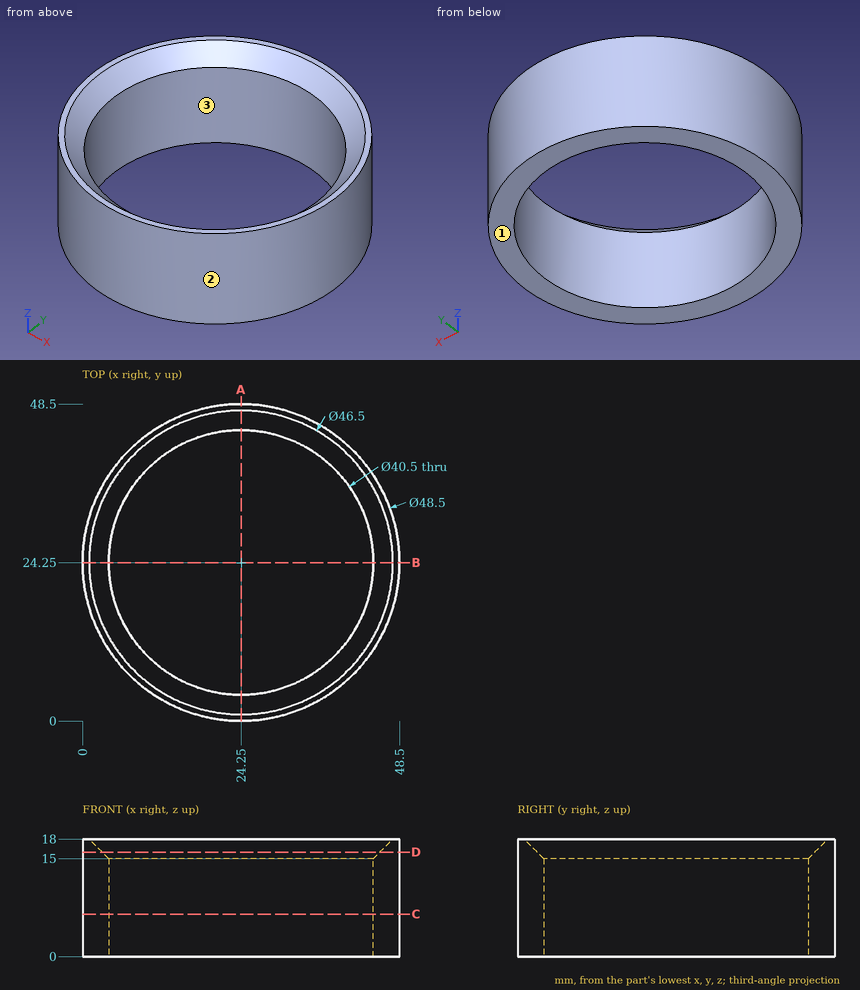
Drawing for the job (mm, zero at the part's lowest x, y, z). Give positions to 0.01 mm unless a question says otherwise; leave off trailing zeros. Order: outer loops, then holes, each group sorted by start corner. A loop starts at its lowest first (then second) coordinate and runs counter-clockwise, first axis right, second up. Notation, with made-up numbers: M -30,53.25 L 17,53.25 A3 cw 17,58.25 Z; hole C -38,29 d2. An arc over 180 degrees is marked long. Put each result on its own line as item: value. Start each with the question number.
(1) Saw through at C-C, the plane z = 6.5. Write the cut outline in (x, y).
(2) Drill centre lines: line 1 along Y through (x, z) = (24.25, 11.5); line 2 along X through (y, z) = (9.5, 4.5). Where is each one in solid material? Low to high.
(3) Flat gauge pins, fed straight in: pin 1 Ø10 at (y, z) = (43, 14) entering from -X (3 decimals); pin 2 Ø8 at (x, z) = (7, 2.5) entering from -Y; pin 3 Ø1 at (x, z) = (43.5, 10) entering from -Y. Where does each tip first touch, or does it go through?
(4) Saw through at D-D, the plane z = 16. Write the cut outline in (x, y).
(5) Saw through at A-A, the plane x = 24.25. Write the cut outline in (y, z).
(6) Mould opens along X. For the marked faces 1, 2 and 3 say: +X half, -X half, draft (parallel to the pull), parting line (faces both ways), or undercut.
Check result:
1. outline: C 24.25,24.25 d48.5; hole C 24.25,24.25 d40.5
2. line 1: y = 0 to 4, 44.5 to 48.5
2. line 2: x = 5 to 10.38, 38.12 to 43.5
3. pin 1: stops at x = 4.275
3. pin 2: stops at y = 3.94
3. pin 3: stops at y = 8.87
4. outline: C 24.25,24.25 d48.5; hole C 24.25,24.25 d42.5
5. outline: M 0,0 L 4,0 L 4,15 L 1,18 L 0,18 Z; M 44.5,0 L 48.5,0 L 48.5,18 L 47.5,18 L 44.5,15 Z
6. face 1: draft
6. face 2: parting line
6. face 3: undercut
